from build123d import *

# Parameters (mm, degrees)
PAD_DEPTH    = 0.34
SKETCH001_W  = 0.156622
SKETCH001_H  = 0.149374
POCKET_DEPTH = 5
POCKET_TAPER = -2


with BuildPart() as part:
    # Sketch → Pad (new body)
    with BuildSketch(Plane.XY):
        with BuildLine():
            Line((0, -4), (0, 0))
            ThreePointArc((-80, 3.226265), (-40.032514, 0.806894), (0, 0))
            ThreePointArc((-80, 3.226265), (-76.048382, 0.88435), (-71.642975, -0.416513))
            ThreePointArc((-71.642975, -0.416513), (-35.876826, -3.314616), (0, -4))
        make_face()
    extrude(amount=PAD_DEPTH)

    # Sketch001 (on Face6 of Pad) → Pocket (cut)
    with BuildSketch(Plane.XY.offset(0.34)):
        with Locations((28.704066, -26.028716)):
            Rectangle(SKETCH001_W, SKETCH001_H)
        with BuildLine():
            ThreePointArc((-4.941031, -1.182712), (-5.617721, -0.719636), (-5.947757, -1.470253))
            Line((-4.911924, -3.539593), (-5.947757, -1.470253))
            Line((-4.911924, -3.539593), (-3.916345, -1.422037))
            ThreePointArc((-3.916345, -1.422037), (-4.280826, -0.669294), (-4.941031, -1.182712))
        make_face()
    extrude(amount=-POCKET_DEPTH, taper=POCKET_TAPER, mode=Mode.SUBTRACT)


solid = part.part
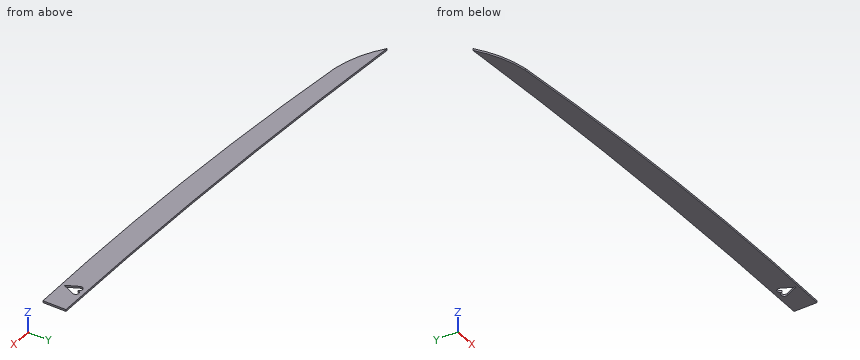
The model under review builds one solid part; all positions refer to its coordinate system, in mm. Round coordinates to 2 decimals unless told otherwise and drop trailing zeros. Loops run counter-clockwise (first coordinate to the right, second up) from the corner with the lowest first, then second, coordinate; pieces in that order, holes last. Notation, with made-up numbers: (40, 28) -> (74, 28) arc R28 cw to (74, 48) -> close; hole circle Ø9 at (10, -16.5). An arc over 180 degrees is marked (long way). Write item = value, one per line. Start each with the question number.
Item 1: Take a section at A-A on x = -68. Give the boundary of the cut face in (y, z), plus the area to 3 significant figures.
Item 2: To check wall thickness, follow L1, parallel to Y at x = -9, z = 0.25; L2, parallel to Y at x = -31.5, z = 0.15. State the ranges of each line that lie inside material, in increasing order.
Item 3: Take a section at B-B on y = 2. Give the boundary of the cut face in (x, z).
Result:
q1.outline = (-0.81, 0) -> (2.33, 0) -> (2.33, 0.34) -> (-0.81, 0.34) -> close
q1.area = 1.07 mm²
q2.L1 = -4.04 to 0.04
q2.L2 = -3.52 to 0.5
q3.outline = (-78.21, 0) -> (-63.01, 0) -> (-63.01, 0.34) -> (-78.21, 0.34) -> close
